from build123d import *

# Parameters (mm, degrees)
BOSS_EXTRUDE1_START = -48
BOSS_EXTRUDE1_DEPTH = 48
SKETCH3_W           = 30
SKETCH3_H           = 10.671288352
SKETCH3_H_2         = 13.328711648
CUT_EXTRUDE1_DEPTH  = 18


# Read off the part's stored shape, not the designer's step: Boss-Extrude1
with BuildPart() as part:
    # Boss-Extrude1 outline → Boss-Extrude1 (new body)
    with BuildSketch(Plane(origin=(0, 0, 0), x_dir=(0, 0, -1), z_dir=(1, 0, 0)).offset(BOSS_EXTRUDE1_START)):
        Polygon((-31.189156063, -12), (-31.189156063, 0), (16.810843937, 0), (16.810843937, -12), (36.810843937, -12), (36.810843937, 0), (22.810843937, 28), (22.810843937, 46), (-37.189156063, 46), (-37.189156063, 28), (-51.189156063, 0), (-51.189156063, -12), align=None)
    extrude(amount=BOSS_EXTRUDE1_DEPTH)

    # Sketch3 → Cut-Extrude1 (cut)
    with BuildSketch(Plane(origin=(0, 46, 0), x_dir=(1, 0, 0), z_dir=(0, 1, 0))):
        with Locations((-24, -31.853511887)):
            Rectangle(SKETCH3_W, SKETCH3_H)
        with Locations((-24, 16.146488113)):
            Rectangle(SKETCH3_W, SKETCH3_H_2)
    extrude(amount=-CUT_EXTRUDE1_DEPTH, mode=Mode.SUBTRACT)


solid = part.part
Check sheet for the modelled part. Datum: model origin and axes. Units: mm. A direction names the side the tool comes from. Round coordinates to 2 decimals unless told otherwise and drop trailing zeros. Order: outer loops, then holes, each group sorted by start corner. A loop starts at its lowest first (then second) coordinate and runs counter-clockwise, first axis right, second up.
(1) Access from +Z, -Z, +X, -X, +Y, -Y to the whole of each face (thin tool, end or side, straight path). Record for faces 1 (the flat face through (-5, 37, 37.189)), 2 (the flat face through (-39, 37, -16)), 3 (the flat face through (-24, 28, 32)).
(2) Cross-section at A-A, the plane y = -1. Enter the section's corners in (x, z).
(3) Draft check along Z on faces 4 (the flat face through (-24, -6, 51.189)), 5 (the flat face through (-24, 0, 8)), 6 (the flat face through (-24.34, 13.8, -29.91)). Enter one of: pulls with the +Z half, pulls with the -Z half, needs draft (parallel to the pull), parting line crosses it, or undercut.
(4) Cross-section at C-C, the plane z = 33. Enter the section's corners in (x, y), and give its area (3 significant figures).
(5) Scan lines: probe 1 along Z at (x, y) = (-5, -2.5); probe 2 along Y at (x, z) = (-21.5, 15); probe 3 along Y at (x, z) = (-22, -12.5). Record each from-to range of solid material in increasing order.
(6) Cross-section at B-B, the plane y = 39. Enter the section's corners in (x, z).
(7) Cross-section at D-D, the plane x = -4. Enter the section's corners in (y, z).
(8) Go/stop test with flat-tipped pins: P1, Ø6, axis at x = -16, y = 9.5, coming from the +Z side; P2, Ø7, axis at x = -4, y = 36, coming from the +Z side; P3, Ø11.5, axis at x = -29, z = 31.5, coming from the +Y side; P4, Ø1, axis at x = -33, y = 5, coming from the +Z side. Record where each tip stops, or that it passes through.
Check sheet entries:
1. face 1: +Z, +X, -X, +Y
1. face 2: -Z, +Y
1. face 3: +Z, +Y
2. outline: (-48, -36.81) - (0, -36.81) - (0, -16.81) - (-48, -16.81) - close; (-48, 31.19) - (0, 31.19) - (0, 51.19) - (-48, 51.19) - close
3. face 4: pulls with the +Z half
3. face 5: undercut
3. face 6: pulls with the -Z half
4. outline: (-48, -12) - (0, -12) - (0, 46) - (-9, 46) - (-9, 28) - (-39, 28) - (-39, 46) - (-48, 46) - close
4. area: 2,240 mm2
5. probe 1: z = -36.81 to -16.81, 31.19 to 51.19
5. probe 2: y = 0 to 46
5. probe 3: y = 0 to 28
6. outline: (-48, -22.81) - (-39, -22.81) - (-39, -9.48) - (-9, -9.48) - (-9, -22.81) - (0, -22.81) - (0, 37.19) - (-9, 37.19) - (-9, 26.52) - (-39, 26.52) - (-39, 37.19) - (-48, 37.19) - close
7. outline: (-12, -36.81) - (0, -36.81) - (28, -22.81) - (46, -22.81) - (46, 37.19) - (28, 37.19) - (0, 51.19) - (-12, 51.19) - (-12, 31.19) - (0, 31.19) - (0, -16.81) - (-12, -16.81) - close
8. P1: stops at z = 47.94
8. P2: stops at z = 37.19
8. P3: stops at y = 46
8. P4: stops at z = 48.94
